CAD build for the part. Positions are in the model's coordinates, mm. Give positions to 0.01 mm unless a question says otherwise; leave off trailing zeros. Loops run counter-clockwise (first coordinate to the right, second up) from the corner with the lowest first, then second, coordinate; pieces in that order, holes last.
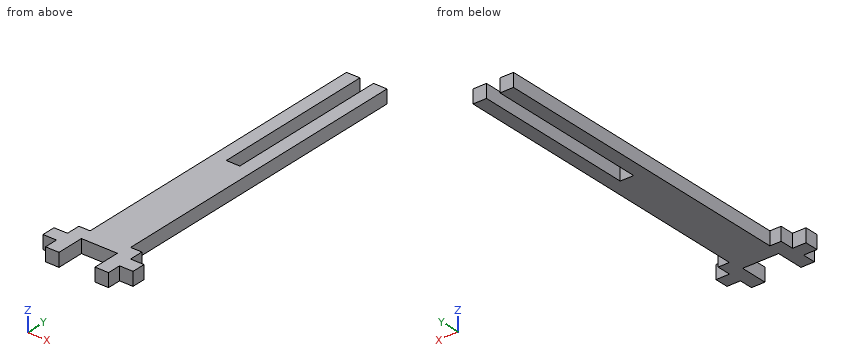
```python
from build123d import *

# Parameters (mm, degrees)
EXTRUDE_1_DEPTH     = 3
SKETCH_2_W          = 3
SKETCH_2_H          = 36.495999937
CUT_EXTRUDE_1_DEPTH = 3
SKETCH_3_W          = 3
SKETCH_3_H          = 3
EXTRUDE_2_DEPTH     = 3


with BuildPart() as part:
    # 스케치1 → 보스-돌출1 (new body)
    with BuildSketch(Plane.XY):
        Polygon((-4.5, 39.545999937), (4.5, 39.545999937), (4.5, -30.445999937), (7, -30.445999937), (7, -39.545999937), (4, -39.545999937), (4, -33.445999937), (-4, -33.445999937), (-4, -39.545999937), (-7, -39.545999937), (-7, -30.445999937), (-4.5, -30.445999937), align=None)
    extrude(amount=EXTRUDE_1_DEPTH)

    # 스케치2 → 컷-돌출1 (cut)
    with BuildSketch(Plane.XY.offset(3)):
        with Locations((0, 21.297999969)):
            Rectangle(SKETCH_2_W, SKETCH_2_H)
    extrude(amount=-CUT_EXTRUDE_1_DEPTH, mode=Mode.SUBTRACT)

    # 스케치3 → 보스-돌출2 (add)
    with BuildSketch(Plane.XY.offset(3)):
        with Locations((-8.5, -35.045999937)):
            Rectangle(SKETCH_3_W, SKETCH_3_H)
        with Locations((8.5, -35.045999937)):
            Rectangle(SKETCH_3_W, SKETCH_3_H)
    extrude(amount=-EXTRUDE_2_DEPTH)


solid = part.part
```
1. Saw through at D-D, the plane y = -3. List the corners of the cut face in (x, z), and give its area (3 significant figures).
Responses:
outline: (-4.5, 0) - (4.5, 0) - (4.5, 3) - (-4.5, 3) - close
area: 27.0 mm2
2. Saw through at B-B, the plane z = 0.9. List the corners of the cut face in (x, y), and give its area (3 significant figures).
Responses:
outline: (-10, -36.55) - (-7, -36.55) - (-7, -39.55) - (-4, -39.55) - (-4, -33.45) - (4, -33.45) - (4, -39.55) - (7, -39.55) - (7, -36.55) - (10, -36.55) - (10, -33.55) - (7, -33.55) - (7, -30.45) - (4.5, -30.45) - (4.5, 39.55) - (1.5, 39.55) - (1.5, 3.05) - (-1.5, 3.05) - (-1.5, 39.55) - (-4.5, 39.55) - (-4.5, -30.45) - (-7, -30.45) - (-7, -33.55) - (-10, -33.55) - close
area: 617 mm2
3. Probe line 1 along X through (y, z) = (34, 2); line 2 along Y through (x, z) = (5.5, 2.7); line 3 along Y through (x, z) = (-8.5, 2.15). List the from-to ranges inside material, lowest first.
Responses:
line 1: x = -4.5 to -1.5, 1.5 to 4.5
line 2: y = -39.55 to -30.45
line 3: y = -36.55 to -33.55
4. Saw through at C-C, the plane x = 5.25. List the corners of the cut face in (y, z).
Responses:
outline: (-39.55, 0) - (-30.45, 0) - (-30.45, 3) - (-39.55, 3) - close
5. Saw through at A-A, the plane y = 13. List the corners of the cut face in (x, z).
Responses:
outline: (-4.5, 0) - (-1.5, 0) - (-1.5, 3) - (-4.5, 3) - close; (1.5, 0) - (4.5, 0) - (4.5, 3) - (1.5, 3) - close
6. Drop flat-ended pins along their axis: pin 1 (0.8 mm diameter, centred on x = 5.5, z = 1, fed in from +Y); pin 2 (12 mm diameter, centred on x = 7.5, y = 13, fed in from +Z); pin 3 (1.5 mm diameter, centred on y = 24, z = 1, fed in from -X); pin 4 (1.5 mm diameter, centred on y = 11.5, z = 1, fed in from +X). Give the stop position or say it passes through.
Responses:
pin 1: stops at y = -30.45
pin 2: stops at z = 3
pin 3: stops at x = -4.5
pin 4: stops at x = 4.5
